```python
from build123d import *

# Parameters (mm, degrees)
F0_W     = 71.12
F0_H     = 61.976
F1_DEPTH = 35.56
F2_W     = 71.12
F2_H     = 10.16
F3_DEPTH = 51.816
F5_DEPTH = 60.961
F6_R     = 19.05
F7_DEPTH = 67.173316


with BuildPart() as f1:
    # F0 (on Front) → F1 (new body, symmetric)
    with BuildSketch(Plane.XZ):
        with Locations((35.56, 30.988)):
            Rectangle(F0_W, F0_H)
    extrude(amount=F1_DEPTH, both=True)

    # F2 (on face) → F3 (cut)
    with BuildSketch(Plane.XY.offset(61.976)):
        with Locations((35.56, -30.48)):
            Rectangle(F2_W, F2_H)
        with Locations((35.56, 30.48)):
            Rectangle(F2_W, F2_H)
    extrude(amount=-F3_DEPTH, mode=Mode.SUBTRACT)

    # F4 (on face) → F5 (cut, through all)
    with BuildSketch(Plane.XZ.offset(25.4)):
        Polygon((0, 61.976), (0, 41.656), (20.32, 61.976), align=None)
        Polygon((71.12, 61.976), (33.02, 61.976), (71.12, 23.876), align=None)
    extrude(amount=-F5_DEPTH, mode=Mode.SUBTRACT)

    # F6 (on face) → F7 (cut, through all)
    with BuildSketch(Plane(origin=(47.498, 0, 47.498), x_dir=(0.707107, 0, -0.707107), z_dir=(0.707107, 0, 0.707107))):
        with Locations((8.006553, 0)):
            Circle(F6_R)
    extrude(amount=-F7_DEPTH, mode=Mode.SUBTRACT)


solid = f1.part
```
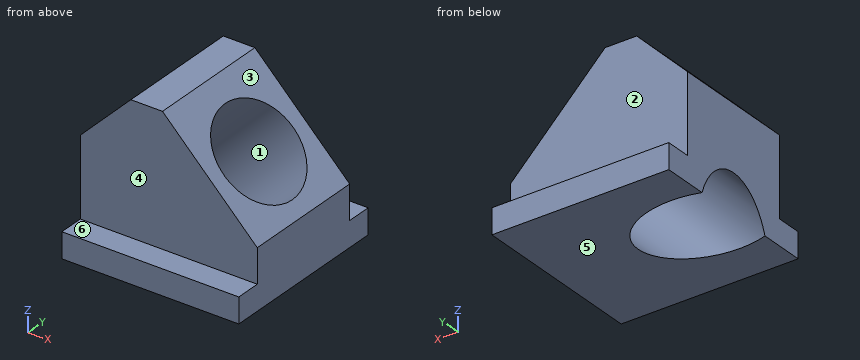
Read the model definition and answer for the solid it produces. Units are mm, in the model's axes. Face numbers are marked on the shaded views. A direction names the side the tool comes from. Coordinates: 2 decimals unless noted, no trailing zeros. Write each loop counter-clockwise with the first axis right and the second up, starting at its lowest first coordinate (ties: lowest second). Pieces come first, ordered by that corner, then holes. Notation, with made-up numbers: (-7.75, -31.5) -> (47.25, -31.5) arc R28 cw to (47.25, 0.5) -> close; hole circle Ø1 at (52.25, 64.5). An arc over 180 degrees is marked (long way). Return JSON: item names as keys, results as strings.
1. A tool of negligible diameter and unlimited length cuts with its end or side. For the marked faces 5 and 6, from which of +Z, -Z, +X, -X, +Y, -Y can it reach the whole face along a straight path? Write none if from no direction.
Found:
{"face 5": "-Z, +X, -X, +Y, -Y", "face 6": "+Z, +X, -X, -Y"}
2. Each of these flat-tipped pins is pushed along its axis until it touches: P1, Ø8, axis at x = 13.5, y = 1.5, coming from the -Z side; P2, Ø1.5, axis at x = 55.5, z = 13.5, coming from the -Y side; P3, Ø1.5, axis at y = -11, z = 24.5, coming from the -X side; P4, Ø6, axis at x = 13, y = -5, coming from the +Z side. Where does it stop, or does it pass through?
Found:
{"P1": "z = 25", "P2": "y = -25.4", "P3": "x = 0", "P4": "z = 57.66"}
3. A cutting plane is placed at A-A (y = 16). Determine the outline of the cut face in (x, z), and give its area (3 significant figures).
Found:
{"outline": "(0, 3.3) -> (45.85, 49.15) -> (33.02, 61.98) -> (20.32, 61.98) -> (0, 41.66) -> close; (25.95, 0) -> (71.12, 0) -> (71.12, 23.88) -> (60.47, 34.53) -> close", "area": "2,260 mm2"}
4. Find the intervals of material crossed by line 1 along Y through (x, z) = (11, 49); line 2 along X through (y, z) = (2.5, 24); line 3 along Y through (x, z) = (9, 14), in increasing order. Write a range as from..to.
Found:
{"line 1": "-25.4..25.4", "line 2": "0..8.62, 62.03..71", "line 3": "-25.4..-15.16, 15.16..25.4"}
5. Determine the mould class of the marked faces 1, 2, 3 and 4 for opening direction Y: pulls with the +Y half, pulls with the -Y half, needs draft (parallel to the pull), parting line crosses it, or undercut.
Found:
{"face 1": "undercut", "face 2": "pulls with the +Y half", "face 3": "needs draft", "face 4": "pulls with the -Y half"}
6. A cutting plane is placed at B-B (y = 2). Determine the outline of the cut face in (x, z).
Found:
{"outline": "(0, 15.47) -> (39.76, 55.23) -> (33.02, 61.98) -> (20.32, 61.98) -> (0, 41.66) -> close; (38.11, 0) -> (71.12, 0) -> (71.12, 23.88) -> (66.56, 28.44) -> close"}
